from build123d import *

# Parameters (mm, degrees)
BOX139_W                    = 15
BOX139_H                    = 21
BOX139_DEPTH                = 23
BOX139_PLACEMENT_ANGLE      = 60
CYLINDER260_R               = 2
CYLINDER260_DEPTH           = 46
CYLINDER260_PLACEMENT_ANGLE = 330
CYLINDER227_R               = 2
CYLINDER227_DEPTH           = 10
CYLINDER227_PLACEMENT_ANGLE = 45
CYLINDER224_R               = 3
CYLINDER224_DEPTH           = 37
CYLINDER222_R               = 0.5
CYLINDER222_DEPTH           = 10
CYLINDER219_R               = 2
CYLINDER219_DEPTH           = 4
CYLINDER223_R               = 3
CYLINDER223_DEPTH           = 10
BOX110_W                    = 10
BOX110_H                    = 10
BOX110_DEPTH                = 10
BOX108_W                    = 2
BOX108_H                    = 10
BOX108_DEPTH                = 10
BOX109_W                    = 10
BOX109_H                    = 10
BOX109_DEPTH                = 10
CYLINDER221_R               = 5
CYLINDER221_DEPTH           = 10
CYLINDER220_R               = 5
CYLINDER220_DEPTH           = 10
BOX101_W                    = 10
BOX101_H                    = 10
BOX101_DEPTH                = 20
BOX101_PLACEMENT_ANGLE      = 330
BOX100_W                    = 12
BOX100_H                    = 10
BOX100_DEPTH                = 17
BOX100_PLACEMENT_ANGLE      = 30
BOX098_W                    = 12.5
BOX098_H                    = 10
BOX098_DEPTH                = 43


with BuildPart() as cube139:
    # Box139 → Box139 (new body)
    with BuildSketch(Plane.XY):
        with Locations((7.5, 10.5)):
            Rectangle(BOX139_W, BOX139_H)
    extrude(amount=BOX139_DEPTH)


with BuildPart() as cube139_1:
    # Box139 placement: moved
    add(cube139.part.moved(Location((-59.2, -11, -91.360962))).rotate(Axis((-59.2, -11, -91.360962), (0, 1, 0)), BOX139_PLACEMENT_ANGLE))


with BuildPart() as cylinder260:
    # Cylinder260 → Cylinder260 (new body)
    with BuildSketch(Plane.XY):
        Circle(CYLINDER260_R)
    extrude(amount=CYLINDER260_DEPTH)


with BuildPart() as cylinder260_1:
    # Cylinder260 placement: moved
    add(cylinder260.part.moved(Location((-50.83, 0, -93.18))).rotate(Axis((-50.83, 0, -93.18), (0, 1, 0)), CYLINDER260_PLACEMENT_ANGLE))


with BuildPart() as cylinder227:
    # Cylinder227 → Cylinder227 (new body)
    with BuildSketch(Plane.XY):
        Circle(CYLINDER227_R)
    extrude(amount=CYLINDER227_DEPTH)


with BuildPart() as cylinder227_1:
    # Cylinder227 placement: moved
    add(cylinder227.part.moved(Location((-62.041631, 0, -84.020815))).rotate(Axis((-62.041631, 0, -84.020815), (0, 1, 0)), CYLINDER227_PLACEMENT_ANGLE))


with BuildPart() as cylinder224:
    # Cylinder224 → Cylinder224 (new body)
    with BuildSketch(Plane(origin=(-52, 0, -84.5), x_dir=(1, 0, 0), z_dir=(0, 0, 1))):
        Circle(CYLINDER224_R)
    extrude(amount=CYLINDER224_DEPTH)


with BuildPart() as cylinder222:
    # Cylinder222 → Cylinder222 (new body)
    with BuildSketch(Plane(origin=(-5, 0, -7), x_dir=(0, 0, -1), z_dir=(1, 0, 0))):
        Circle(CYLINDER222_R)
    extrude(amount=CYLINDER222_DEPTH)


with BuildPart() as cylinder219:
    # Cylinder219 → Cylinder219 (new body)
    with BuildSketch(Plane(origin=(-2, -50, 1), x_dir=(0, 0, -1), z_dir=(1, 0, 0))):
        Circle(CYLINDER219_R)
    extrude(amount=CYLINDER219_DEPTH)


with BuildPart() as cylinder223:
    # Cylinder223 → Cylinder223 (new body)
    with BuildSketch(Plane(origin=(0, -50, -12), x_dir=(1, 0, 0), z_dir=(0, 0, 1))):
        Circle(CYLINDER223_R)
    extrude(amount=CYLINDER223_DEPTH)


with BuildPart() as cube110:
    # Box110 → Box110 (new body)
    with BuildSketch(Plane(origin=(-12, -55, -2), x_dir=(1, 0, 0), z_dir=(0, 0, 1))):
        with Locations((5, 5)):
            Rectangle(BOX110_W, BOX110_H)
    extrude(amount=BOX110_DEPTH)


with BuildPart() as cube108:
    # Box108 → Box108 (new body)
    with BuildSketch(Plane(origin=(-1, -55, -2), x_dir=(1, 0, 0), z_dir=(0, 0, 1))):
        with Locations((1, 5)):
            Rectangle(BOX108_W, BOX108_H)
    extrude(amount=BOX108_DEPTH)


with BuildPart() as cube109:
    # Box109 → Box109 (new body)
    with BuildSketch(Plane(origin=(2, -55, -2), x_dir=(1, 0, 0), z_dir=(0, 0, 1))):
        with Locations((5, 5)):
            Rectangle(BOX109_W, BOX109_H)
    extrude(amount=BOX109_DEPTH)


with BuildPart() as cylinder221:
    # Cylinder221 → Cylinder221 (new body)
    with BuildSketch(Plane(origin=(0, -50, -10), x_dir=(1, 0, 0), z_dir=(0, 0, 1))):
        Circle(CYLINDER221_R)
    extrude(amount=CYLINDER221_DEPTH)


with BuildPart() as sphere045:
    # Sphere045 → Sphere045 (revolve)
    with BuildSketch(Plane.XZ.offset(50)):
        with BuildLine():
            ThreePointArc((5, 0), (3.535534, 3.535534), (0, 5))
            Line((0, 5), (0, 0))
            Line((0, 0), (5, 0))
        make_face()
    revolve(axis=Axis((0, -50, 0), (0, 0, 1)))


with BuildPart() as cut204006013:
    # Cylinder220 → Cylinder220 (new body)
    with BuildSketch(Plane(origin=(0, -50, -7), x_dir=(1, 0, 0), z_dir=(0, 0, 1))):
        Circle(CYLINDER220_R)
    extrude(amount=CYLINDER220_DEPTH)

    # Common038: intersect Sphere045
    add(sphere045.part, mode=Mode.INTERSECT)

    # Fusion005077020006: union Cylinder221
    add(cylinder221.part)

    # Cut204006012: cut Cube109
    add(cube109.part, mode=Mode.SUBTRACT)

    # Cut204006014: cut Cube108
    add(cube108.part, mode=Mode.SUBTRACT)

    # Cut204006015: cut Cube110
    add(cube110.part, mode=Mode.SUBTRACT)

    # Cut204006011: cut Cylinder223
    add(cylinder223.part, mode=Mode.SUBTRACT)

    # Fusion005077020005: union Cylinder219
    add(cylinder219.part)


with BuildPart() as cut204006013_1:
    # Fusion005077020007 placement: moved
    add(cut204006013.part.moved(Location((0, 50, -8.5))))

    # Cut204006013: cut Cylinder222
    add(cylinder222.part, mode=Mode.SUBTRACT)


with BuildPart() as cut204006013_2:
    # Cut204006013 placement: moved
    add(cut204006013_1.part.moved(Location((-52, 0, -37))))


with BuildPart() as cube101:
    # Box101 → Box101 (new body)
    with BuildSketch(Plane.XY):
        with Locations((5, 5)):
            Rectangle(BOX101_W, BOX101_H)
    extrude(amount=BOX101_DEPTH)


with BuildPart() as cube101_1:
    # Box101 placement: moved
    add(cube101.part.moved(Location((-168.49167, -5, -108.102886))).rotate(Axis((-168.49167, -5, -108.102886), (0, 1, 0)), BOX101_PLACEMENT_ANGLE))


with BuildPart() as cube100:
    # Box100 → Box100 (new body)
    with BuildSketch(Plane.XY):
        with Locations((6, 5)):
            Rectangle(BOX100_W, BOX100_H)
    extrude(amount=BOX100_DEPTH)


with BuildPart() as cube100_1:
    # Box100 placement: moved
    add(cube100.part.moved(Location((-167.14, -5, -90.45))).rotate(Axis((-167.14, -5, -90.45), (0, -1, 0)), BOX100_PLACEMENT_ANGLE))


with BuildPart() as cut204006069001:
    # Box098 → Box098 (new body)
    with BuildSketch(Plane(origin=(-168, -5, -90.5), x_dir=(1, 0, 0), z_dir=(0, 0, 1))):
        with Locations((6.25, 5)):
            Rectangle(BOX098_W, BOX098_H)
    extrude(amount=BOX098_DEPTH)

    # Fusion005077020: union Cube100
    add(cube100_1.part)

    # Cut204006: cut Cube101
    add(cube101_1.part, mode=Mode.SUBTRACT)


with BuildPart() as cut204006069001_1:
    # Cut204006001 placement: moved
    add(cut204006069001.part.moved(Location((110, 0, 0))))

    # Fusion005077020009: union Cut204006013
    add(cut204006013_2.part)

    # Cut204006018: cut Cylinder224
    add(cylinder224.part, mode=Mode.SUBTRACT)

    # Cut204006019: cut Cylinder227
    add(cylinder227_1.part, mode=Mode.SUBTRACT)

    # Cut204006067: cut Cylinder260
    add(cylinder260_1.part, mode=Mode.SUBTRACT)

    # Cut204006069: cut Cube139
    add(cube139_1.part, mode=Mode.SUBTRACT)


solid = cut204006069001_1.part
The listing builds one solid part. Answer for the finished solid, in the listing's coordinates (mm). A direction names the side the tool comes from. Coordinates: 2 decimals unless noted, no trailing zeros. Loops run counter-clockwise (first coordinate to the right, second up) from the corner with the lowest first, then second, coordinate; pieces in that order, holes last. Notation, with made-up numbers: (-21, 38) -> (6, 38) arc R10 cw to (6, 49) -> close; hole circle Ø7 at (3, 70.25). An arc over 180 degrees is marked (long way). Write item = value, one per line. Start each with the question number.
1) A cutting plane is placed at A-A (z = -47). Give the vertices of the cut face in (x, y), then the cut area to 3 significant figures.
2) A cutting plane is placed at B-B (z = -55). Give the vertices of the cut face in (x, y).
3) Straight lines are drawn through the part: line 1 (Z direction, x = -50.85, y = 0); line 2 (Y direction, x = -52, z = -70.5); line 3 (X direction, y = 0, z = -75). For each, find the intervals that lie inside material, in ascending order. Write a range as from..to.
4) Given pin 1 Ø2.5 at (y, z) = (1, -45) entering from +X; pin 2 Ø0.5 at (x, y) = (-53.5, 0.5) entering from -Z; pin 3 Ø1.5 at (y, z) = (1, -68.5) entering from -X, each flat-ended and moving along its own axis, determine where each tip first touches the part or whether it passes through.
5) The mould has two halves that part along Y. Classify faces 6 (the face through (-49, -1, -47.5)), 7 (the face through (-52, 0, -43.5)), 8 (the face through (-53, -5, -69)): released by +Y, released by -Y, zero draft, split by the parting line, or undercut.
6) A cutting plane is placed at D-D (x = -47). Give the vertices of the cut face in (y, z), then the cut area to 3 significant figures.
7) A cutting plane is placed at C-C (x = -49.5). Give the vertices of the cut face in (y, z), then the cut area to 3 significant figures.
8) A tool of negligible diameter and unlimited length cuts with its end or side. For faces 1 (the face through (-45.5, 0, -66)), 2 (the face through (-55.4, 0.03, -76.52)), 3 (the face through (-50.5, 0.1, -42.5)), 4 (the face through (-50.5, -4.77, -46.51)), 5 (the face through (-58, 0, -60)), from which of +Z, -Z, +X, -X, +Y, -Y can it reach the whole face along a straight path? Write none if from no direction.
Responses:
q1.outline = (-54, -4.58) arc R5 ccw to (-53, -4.9) -> (-53, 4.9) arc R5 ccw to (-54, 4.58) -> close; (-51, -4.9) arc R5 ccw to (-50, -4.58) -> (-50, 4.58) arc R5 ccw to (-51, 4.9) -> close
q1.area = 19.0 mm²
q2.outline = (-58, -5) -> (-45.5, -5) -> (-45.5, 5) -> (-58, 5) -> close; hole circle Ø6 at (-52, 0)
q3.line_1 = -86.54..-84.5, -47.5..-44.5, -43.5..-42.5
q3.line_2 = -5..-3, 3..5
q3.line_3 = -64.38..-63.64, -59.02..-55, -49..-45.5
q4.pin_1 = -50
q4.pin_2 = -85.14
q4.pin_3 = -58
q5.face_6 = zero draft
q5.face_7 = undercut
q5.face_8 = released by -Y
q6.outline = (-5, -84.32) -> (5, -84.32) -> (5, -47.5) -> (-5, -47.5) -> close
q6.area = 368 mm²
q7.outline = (-5, -85.76) -> (5, -85.76) -> (5, -47.5) -> (1.66, -47.5) -> (1.66, -84.5) -> (-1.66, -84.5) -> (-1.66, -47.5) -> (-5, -47.5) -> close
q7.area = 260 mm²
q8.face_1 = +Z, -Z, +X, +Y, -Y
q8.face_2 = none
q8.face_3 = +Z, +X, -X, +Y, -Y
q8.face_4 = +Z, +X, -Y
q8.face_5 = +Z, -X, +Y, -Y
